Design review of the part built by this model. Coordinates are the model's own, in mm. A direction names the side the tool comes from. Round coordinates to 2 decimals unless told otherwise and drop trailing zeros. Write item = value, one per line.
Autodesk Inventor part; units mm, degrees
ref_plane "YZ Plane" through (0, 0, 0) normal (1, 0, 0) x (0, 1, 0)
ref_plane "XZ Plane" through (0, 0, 0) normal (0, 1, 0) x (-1, 0, 0)
ref_plane "XY Plane" through (0, 0, 0) normal (0, 0, 1) x (1, 0, 0)
ref_plane "Work Plane1" through (0, 0, 0) normal (0, 0, 1) x (1, 0, 0)
sketch "Sketch1" plane through (0, 0, 0) normal (0, 0, 1) x (1, 0, 0)
  circle A0 centre (-23, 51) radius 1.45
  circle A1 centre (-22.4561, -50.4561) radius 1.45
  arc A2 (-27, -50) -> (-22, -55) centre (-22, -50) ccw
  line L0 (-22, -55) -> (22, -55)
  arc A3 (22, -55) -> (27, -50) centre (22, -50) ccw
  line L1 (27, -50) -> (27, 50)
  arc A4 (27, 50) -> (22, 55) centre (22, 50) ccw
  line L2 (22, 55) -> (-22, 55)
  arc A5 (-22, 55) -> (-27, 50) centre (-22, 50) ccw
  line L3 (-27, 50) -> (-27, -50)
  line L4 (-22, 53) -> (22, 53)
  arc A6 (25, 50) -> (22, 53) centre (22, 50) ccw
  line L5 (25, 50) -> (25, -50)
  arc A7 (22, -53) -> (25, -50) centre (22, -50) ccw
  line L6 (22, -53) -> (-22, -53)
  arc A8 (-22, -53) -> (-25, -50) centre (-22.4561, -50.4561) ccw
  line L7 (-25, -50) -> (-25, 50)
  arc A9 (-25, 50) -> (-22, 53) centre (-23, 51) ccw
  point P0 (0, 0)
extrude "Extrusion1" add sketch "Sketch1" along normal blind 4 contours L3 A5 L2 A4 L1 A3 L0 A2 | L4 A6 L5 A7 L6 A8 L7 A9
sketch "Sketch2" plane through (0, 0, 0) normal (0, 0, -1) x (-1, 0, 0)
  line L0 (-25, 50) -> (-25, -50)
  line L1 (-25, 50) -> (-21, 50)
  line L2 (-21, 50) -> (-21, -50)
  line L3 (-21, -50) -> (-25, -50)
  line L4 (-25, -50) -> (-25, 50)
  line L5 (-21, 50) -> (-25, 50)
  line L6 (-25, 50) -> (-25, 51.5)
  line L7 (-25, 51.5) -> (-21, 51.5)
  line L8 (-21, 51.5) -> (-21, 50)
  line L9 (-21, -50) -> (-25, -50)
  line L10 (-25, -50) -> (-25, -51.5)
  line L11 (-25, -51.5) -> (-21, -51.5)
  line L12 (-21, -51.5) -> (-21, -50)
  point P0 (0, 0)
  dimension "d2" = 4
  dimension "d15" = 1.5
  dimension "d16" = 1.5
extrude "Extrusion2" cut sketch "Sketch2" against normal blind 2
sketch "Sketch3" plane through (0, 0, 4) normal (0, 0, 1) x (1, 0, 0)
  line L0 (21, 50) -> (21, -50)
  line L1 (-20, 46) -> (21, 46)
  line L2 (21, 46) -> (21, 43)
  line L3 (21, 43) -> (-20, 43)
  line L4 (-20, 43) -> (-20, 46)
  line L5 (21, 33.3) -> (-20, 33.3)
  line L6 (-20, 36.3) -> (21, 36.3)
  line L7 (21, 36.3) -> (21, 33.3)
  line L8 (-20, 33.3) -> (-20, 36.3)
  line L9 (21, 23.6) -> (-20, 23.6)
  line L10 (-20, 26.6) -> (21, 26.6)
  line L11 (21, 26.6) -> (21, 23.6)
  line L12 (-20, 23.6) -> (-20, 26.6)
  line L13 (21, 13.9) -> (-20, 13.9)
  line L14 (-20, 16.9) -> (21, 16.9)
  line L15 (21, 16.9) -> (21, 13.9)
  line L16 (-20, 13.9) -> (-20, 16.9)
  line L17 (21, 4.2) -> (-20, 4.2)
  line L18 (-20, 7.2) -> (21, 7.2)
  line L19 (21, 7.2) -> (21, 4.2)
  line L20 (-20, 4.2) -> (-20, 7.2)
  line L21 (21, -5.5) -> (-20, -5.5)
  line L22 (-20, -2.5) -> (21, -2.5)
  line L23 (21, -2.5) -> (21, -5.5)
  line L24 (-20, -5.5) -> (-20, -2.5)
  line L25 (21, -15.2) -> (-20, -15.2)
  line L26 (-20, -12.2) -> (21, -12.2)
  line L27 (21, -12.2) -> (21, -15.2)
  line L28 (-20, -15.2) -> (-20, -12.2)
  line L29 (21, -24.9) -> (-20, -24.9)
  line L30 (-20, -21.9) -> (21, -21.9)
  line L31 (21, -21.9) -> (21, -24.9)
  line L32 (-20, -24.9) -> (-20, -21.9)
  line L33 (21, -34.6) -> (-20, -34.6)
  line L34 (-20, -31.6) -> (21, -31.6)
  line L35 (21, -31.6) -> (21, -34.6)
  line L36 (-20, -34.6) -> (-20, -31.6)
  line L37 (21, -44.3) -> (-20, -44.3)
  line L38 (-20, -41.3) -> (21, -41.3)
  line L39 (21, -41.3) -> (21, -44.3)
  line L40 (-20, -44.3) -> (-20, -41.3)
  line L41 (22, 55) -> (-22, 55)
  point P0 (0, 0)
  point P1 (21, -41.3)
  point P2 (21, -31.6)
  point P3 (21, -21.9)
  point P4 (21, -12.2)
  point P5 (21, -2.5)
  point P6 (21, 7.2)
  point P7 (21, 16.9)
  point P8 (21, 26.6)
  point P9 (21, 36.3)
  point P10 (21, 46)
  dimension "d5" = 3
  dimension "d8" = 9.7
  dimension "d17" = 9
extrude "Extrusion3" cut sketch "Sketch3" against normal through all
properties part number "00_Case_Powersupply_Galvo_lid"
1) To check wall thickness, follow L1, parallel to X at y = -30.5, z = 1.95; L2, parallel to Y at x = -23, z = 1.75; L3, parallel to X at y = -41.5, z = 2.95. State the ranges of each line that lie inside material, in increasing order. Write a range as from..to.
Findings:
L1 = -27..21, 25..27
L2 = -54.9..-51.8, -49.11..49.55, 52.45..54.9
L3 = -27..-20, 21..27
2) For faces 3 (the flat face through (0, -41.3, 2)), 4 (the flat face through (21, -38, 1)), list the 3-axis set-ups (+Z, -Z, +X, -X, +Y, -Y) from which the entire face can be reached by the end or side of a thin tool; tool diameter is ignored.
Findings:
face_3 = +Z, -Z
face_4 = -Z
3) The part is to be moulded in two halves that separate along X. For faces 1 (the flat face through (-6, 1, 0)), 2 (the flat face through (-20, -14, 2)), say which applies: released by +X, released by -X, zero draft, split by the parting line, or undercut.
Findings:
face_1 = zero draft
face_2 = undercut
4) We need section A-A on x = 2.5. Give the number of separate pieces and of enclosed holes in the cut face, and give its area (3 significant figures).
Findings:
separate_pieces = 11
enclosed_holes = 0
area = 320 mm^2
